```python
from build123d import *

# Parameters (mm, degrees)
F1_DEPTH       = 127
F2_DEPTH       = 25.4
F5_D           = 6.7564
F5_DEPTH       = 76.2
F5_TIP         = 2.0298273432
F5_ON_F3_D     = 6.7564
F5_ON_F3_DEPTH = 76.2
F5_ON_F3_TIP   = 2.0298273432


with BuildPart() as f1:
    # F0 (on Right) → F1 (new body)
    with BuildSketch(Plane.YZ):
        Polygon((-56.4980393835, 48.746819774), (-59.6730393835, 48.746819774), (-59.6730393835, 23.346819774), (-34.2730393835, 23.346819774), (-34.2730393835, 26.521819774), (-56.4980393835, 26.521819774), align=None)
    extrude(amount=F1_DEPTH)

    # F2 (add): a face of the model
    f2_faces = [f1.faces().sort_by_distance(p)[0] for p in [
        (0, -58.0855393835, 48.3876095291),
    ]]
    extrude(f2_faces, amount=F2_DEPTH)

    # F5
    with Locations(Plane(origin=(0, 0, 23.346819774), x_dir=(1, 0, 0), z_dir=(0, 0, -1))):
        with Locations((114.3, 46.9730393835), (63.5, 46.9730393835), (38.1, 46.9730393835), (12.7, 46.9730393835), (-12.7, 46.9730393835)):
            Hole(F5_D / 2, depth=F5_DEPTH)
            with Locations((0, 0, -(F5_DEPTH + F5_TIP / 2))):  # 118° drill point
                Cone(0, F5_D / 2, F5_TIP, mode=Mode.SUBTRACT)

    # F5 on F3
    with Locations(Plane.XZ.offset(59.6730393835)):
        with Locations((114.3, 36.046819774), (63.5, 36.046819774), (38.1, 36.046819774), (12.7, 36.046819774), (-12.7, 36.046819774)):
            Hole(F5_ON_F3_D / 2, depth=F5_ON_F3_DEPTH)
            with Locations((0, 0, -(F5_ON_F3_DEPTH + F5_ON_F3_TIP / 2))):  # 118° drill point
                Cone(0, F5_ON_F3_D / 2, F5_ON_F3_TIP, mode=Mode.SUBTRACT)


solid = f1.part
```
Model file for the job. Use its own axes, mm. A direction names the side the tool comes from. Round coordinates to 2 decimals unless told otherwise and drop trailing zeros. Loops run counter-clockwise (first coordinate to the right, second up) from the corner with the lowest first, then second, coordinate; pieces in that order, holes last. Notation, with made-up numbers: M 53,14.5 L 60,14.5 A5 ccw 60,20.5 Z; hole C 28.5,47.25 d11. An arc over 180 degrees is marked long. Put each result on its own line as item: value. Start each with the question number.
Item 1: Cut at B-B (y = -37.75). List the corners of the cut face in (x, z).
Item 2: Drill centre lines: line 1 along Y through (x, z) = (-12.7, 24.2); line 2 along Z through (x, y) = (63.5, -59); line 3 along X through (y, z) = (-45, 26). Where is each one in solid material? Low to high.
Item 3: Cut at A-A (x = 63.5). List the corners of the cut face in (y, z), then the cut area to 3 significant figures.
Item 4: Mould opens along Z. For faces 3 (the face through (127, -53, 26)), 4 (the face through (52, -45, 26.522)), 5 (the face through (111.078, -58.063, 37.062)), 6 (the face through (-10.21, -58.06, 38.33)) say: released by +Z, released by -Z, zero draft, split by the parting line, or undercut.
Item 5: Drop flat-ended pins along their axis: P1, Ø11, axis at x = 73.5, z = 34.5, coming from the +Y side; P2, Ø1.5, axis at x = 105.5, y = -49.5, coming from the +Z side; P3, Ø8, axis at x = 63.5, z = 36.05, coming from the -Y side. Give the stop position or say it passes through.
Item 6: Cut at C-C (x = 39.5). List the corners of the cut face in (y, z), then the cut area to 3 significant figures.
Item 7: 3-axis set-ups, long thin cutter, end or side, ignore diameter. For faces 1 (the face through (41.475, -58.063, 36.195)), 2 (the face through (52, -56.498, 37)): which of +Z, -Z, +X, -X, +Y, -Y reach the whole face in a straight line?
Answer block:
1. outline: M -25.4,23.35 L 127,23.35 L 127,26.52 L -25.4,26.52 Z
2. line 1: -59.67 to -50.35, -43.59 to -34.27
2. line 2: 23.35 to 32.67, 39.43 to 48.75
2. line 3: -25.4 to -15.44, -9.96 to 9.96, 15.44 to 35.36, 40.84 to 60.76, 66.24 to 111.56, 117.04 to 127
3. outline: M -59.67,23.35 L -50.35,23.35 L -50.35,26.52 L -56.5,26.52 L -56.5,32.67 L -59.67,32.67 Z; M -59.67,39.43 L -56.5,39.43 L -56.5,48.75 L -59.67,48.75 Z; M -43.59,23.35 L -34.27,23.35 L -34.27,26.52 L -43.59,26.52 Z
3. area: 108 mm2
4. face 3: zero draft
4. face 4: released by +Z
4. face 5: undercut
4. face 6: undercut
5. P1: y = -56.5
5. P2: z = 26.52
5. P3: y = -59.67
6. outline: M -59.67,23.35 L -50.05,23.35 L -50.05,26.52 L -56.5,26.52 L -56.5,32.97 L -59.67,32.97 Z; M -59.67,39.12 L -56.5,39.12 L -56.5,48.75 L -59.67,48.75 Z; M -43.9,23.35 L -34.27,23.35 L -34.27,26.52 L -43.9,26.52 Z
6. area: 112 mm2
7. face 1: +Y, -Y
7. face 2: +Z, +X, -X, +Y
